Answer from the drawing. Dimensions are ordinates in mm from the lowest x, y and z of the part. A direction names the side the tool comes from. Coordinates: 2 decimals unless noted, no trailing zeros. Order: outer loops, then holes, each group sorted by start corner. A loop starts at its lowest first (then second) coordinate and runs counter-clockwise, first axis right, second up. Notation, with made-up numbers: (54, 46) - (110, 46) arc R18 cw to (110, 56) - close; hole circle Ø8 at (74.5, -3). An arc over 180 degrees is marked (long way). Use a Markdown table: item, result. Add a question column.
Item 1: Flat-ended cylindrical pins translate along their axes: P1, Ø1.2, axis at y = 8.5, z = 2.5, coming from the -X side; P2, Ø3, axis at x = 34, y = 10, coming from the +Z side; P3, Ø12.5, axis at y = 27.5, z = 16.5, coming from the -X side. Find the tip coordinate at first contact, or state that the pin passes through.
Item 2: The part is cut by section C-C, the plane z = 8.5. Give the vertices of the cut face in (x, y), then the cut area to 3 significant figures.
Item 3: The part is cut by section B-B, the plane y = 11. Give the vertices of the cut face in (x, z), then the cut area to 3 significant figures.
Item 4: The part is cut by section A-A, the plane z = 19.75. Give the vertices of the cut face in (x, y).
Item 5: The mould has two halves that part along X. Classify the marked faces 4, 5 and 6: released by +X, released by -X, zero draft, split by the parting line, or undercut.
Item 6: The part is cut by section D-D, the plane x = 57. Give the vertices of the cut face in (y, z), then the cut area to 3 significant figures.
Item 7: Find the intervals of material crossed by line 1 along X through (y, z) = (15, 7.75); line 2 along Y through (x, z) = (7, 23.75); line 3 along X through (y, z) = (32.5, 3.5) (1 decimal), in increasing order.
Item 8: For the marked faces 1, 2 and 3, determine the directions among +Z, -Z, +X, -X, +Y, -Y from which every point of the face is accessible in a straight line to the end or side of a thin tool.
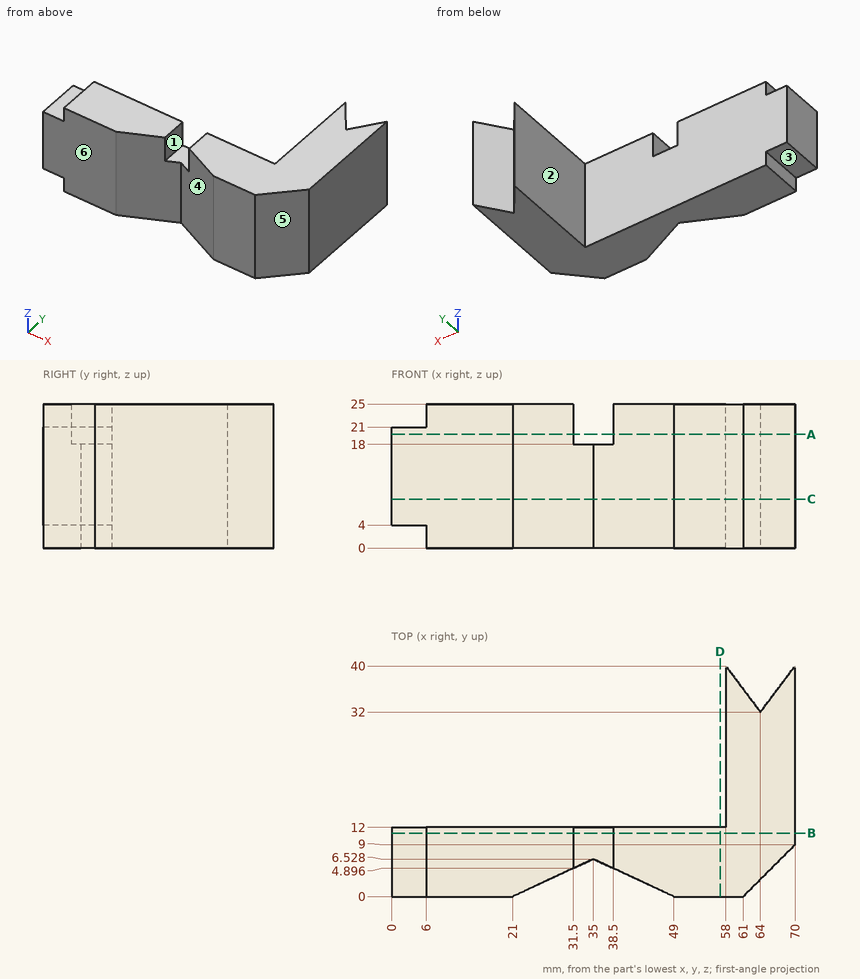
Solution:
| question | item | result |
|---|---|---|
| 1 | P1 | stops at x = 6 |
| 1 | P2 | stops at z = 18 |
| 1 | P3 | stops at x = 58 |
| 2 | outline | (0, 0) - (21, 0) - (35, 6.53) - (49, 0) - (61, 0) - (70, 9) - (70, 40) - (64, 32) - (58, 40) - (58, 12) - (0, 12) - close |
| 2 | area | 996 mm2 |
| 3 | outline | (0, 4) - (6, 4) - (6, 0) - (70, 0) - (70, 25) - (38.5, 25) - (38.5, 18) - (31.5, 18) - (31.5, 25) - (6, 25) - (6, 21) - (0, 21) - close |
| 3 | area | 1,650 mm2 |
| 4 | outline | (0, 0) - (21, 0) - (31.5, 4.9) - (31.5, 12) - (0, 12) - close; (38.5, 4.9) - (49, 0) - (61, 0) - (70, 9) - (70, 40) - (64, 32) - (58, 40) - (58, 12) - (38.5, 12) - close |
| 5 | face 4 | undercut |
| 5 | face 5 | released by +X |
| 5 | face 6 | zero draft |
| 6 | outline | (0, 0) - (12, 0) - (12, 25) - (0, 25) - close |
| 6 | area | 300 mm2 |
| 7 | line 1 | x = 58 to 70 |
| 7 | line 2 | y = 0 to 12 |
| 7 | line 3 | x = 58 to 63.6, 64.4 to 70 |
| 8 | face 1 | +Z, +Y, -Y |
| 8 | face 2 | +Z, -Z, -X, +Y |
| 8 | face 3 | -Z, -X, +Y, -Y |
